from build123d import *

# Parameters (mm, degrees)
SKETCH1_W                                    = 147
SKETCH1_H                                    = 50
BOSS_EXTRUDE1_DEPTH                          = 30
FILLET1_R                                    = 10
SHELL1_T                                     = -3
CUT_EXTRUDE1_DEPTH                           = 3
CSK_FOR_M4_COUNTERSUNK_FLAT_HEAD_SCR_2_COUNT = 2
CSK_FOR_M4_COUNTERSUNK_FLAT_HEAD_SCR_2_PITCH = 32
CSK_FOR_M4_COUNTERSUNK_FLAT_HEAD_SCR_3_COUNT = 2
CSK_FOR_M4_COUNTERSUNK_FLAT_HEAD_SCR_3_PITCH = 64
CUT_EXTRUDE2_REACH                           = 32
SKETCH5_R                                    = 10


with BuildPart() as part:
    # Sketch1 → Boss-Extrude1 (new body)
    with BuildSketch(Plane(origin=(0, 0, 0), x_dir=(1, 0, 0), z_dir=(0, 1, 0))):
        Rectangle(SKETCH1_W, SKETCH1_H)
    extrude(amount=BOSS_EXTRUDE1_DEPTH)

    # Fillet1
    fillet1_edges = [part.edges().sort_by_distance(p)[0] for p in [
        (0, 0, -25),
        (0, 30, -25),
    ]]
    fillet(fillet1_edges, radius=FILLET1_R)

    # Shell1
    shell1_openings = [part.faces().sort_by_distance(p)[0] for p in [
        (0, 15, 25),
    ]]
    offset(amount=SHELL1_T, openings=shell1_openings, kind=Kind.INTERSECTION)

    # Sketch2 → Cut-Extrude1 (cut)
    with BuildSketch(Plane(origin=(0, 30, 0), x_dir=(1, 0, 0), z_dir=(0, 1, 0))):
        with BuildLine():
            Line((-70.5, -25), (-70.5, 5))
            ThreePointArc((-70.5, 5), (-67.5, 8), (-64.5, 5))
            Line((-64.5, 5), (-64.5, -25))
            Line((-64.5, -25), (-70.5, -25))
        make_face()
    cut_extrude1 = extrude(amount=-CUT_EXTRUDE1_DEPTH, mode=Mode.SUBTRACT)

    # Mirror1: Cut-Extrude1 across plane
    add(cut_extrude1.mirror(Plane(origin=(0, 0, 0), x_dir=(0, 0, 1), z_dir=(1, 0, 0))), mode=Mode.SUBTRACT)

    # Sketch3 → CSK for M4 Countersunk Flat Head Screw1 (revolve, cut)
    with BuildSketch(Plane(origin=(-32, 27, 0), x_dir=(0, 0, -1), z_dir=(1, 0, 0))):
        Polygon((0, 0), (0, 3), (2.25, 3), (2.25, 2.45), (4.7, 0), align=None)
    csk_for_m4_countersunk_flat_head_screw1 = revolve(axis=Axis((-32, 20.65, 0), (0, 1, 0)), mode=Mode.SUBTRACT)

    # CSK for M4 Countersunk Flat Head Scr 2: CSK for M4 Countersunk Flat Head Screw1 ×2
    with Locations(*[(i * CSK_FOR_M4_COUNTERSUNK_FLAT_HEAD_SCR_2_PITCH, 0, 0) for i in range(1, CSK_FOR_M4_COUNTERSUNK_FLAT_HEAD_SCR_2_COUNT)]):
        add(csk_for_m4_countersunk_flat_head_screw1, mode=Mode.SUBTRACT)

    # CSK for M4 Countersunk Flat Head Scr 3: CSK for M4 Countersunk Flat Head Screw1 ×2
    with Locations(*[(i * CSK_FOR_M4_COUNTERSUNK_FLAT_HEAD_SCR_3_PITCH, 0, 0) for i in range(1, CSK_FOR_M4_COUNTERSUNK_FLAT_HEAD_SCR_3_COUNT)]):
        add(csk_for_m4_countersunk_flat_head_screw1, mode=Mode.SUBTRACT)

    # Sketch5 → Cut-Extrude2 (cut, up to next)
    with BuildSketch(Plane.XZ, mode=Mode.PRIVATE) as cut_extrude2_sk1:
        Circle(SKETCH5_R)
    cut_extrude2_tool1 = extrude(cut_extrude2_sk1.sketch, amount=-CUT_EXTRUDE2_REACH, mode=Mode.PRIVATE) & part.part
    add(cut_extrude2_tool1.solids().sort_by_distance((0, 0, 0))[0], mode=Mode.SUBTRACT)
    # Sketch5 → Cut-Extrude2 (cut, up to next)
    with BuildSketch(Plane.XZ, mode=Mode.PRIVATE) as cut_extrude2_sk2:
        with Locations((-32, 0)):
            Circle(SKETCH5_R)
    cut_extrude2_tool2 = extrude(cut_extrude2_sk2.sketch, amount=-CUT_EXTRUDE2_REACH, mode=Mode.PRIVATE) & part.part
    add(cut_extrude2_tool2.solids().sort_by_distance((-32, 0, 0))[0], mode=Mode.SUBTRACT)
    # Sketch5 → Cut-Extrude2 (cut, up to next)
    with BuildSketch(Plane.XZ, mode=Mode.PRIVATE) as cut_extrude2_sk3:
        with Locations((32, 0)):
            Circle(SKETCH5_R)
    cut_extrude2_tool3 = extrude(cut_extrude2_sk3.sketch, amount=-CUT_EXTRUDE2_REACH, mode=Mode.PRIVATE) & part.part
    add(cut_extrude2_tool3.solids().sort_by_distance((32, 0, 0))[0], mode=Mode.SUBTRACT)


solid = part.part
Work out the finished part from the listing and answer in its coordinate system (mm). A direction names the side the tool comes from. Give positions to 0.01 mm unless a question says otherwise; leave off trailing zeros. Write each loop counter-clockwise with the first axis right and the second up, starting at its lowest first coordinate (ties: lowest second). Pieces come first, ordered by that corner, then holes.
Q1. The part is cut by section C-C on x = 67.5. Give the vertices of the cut face in (y, z), and give its area (3 significant figures).
Answer:
outline: (0, -15) arc R10 ccw to (10, -25) - (20, -25) arc R10 ccw to (30, -15) - (30, -8) - (27, -8) - (27, -15) arc R7 cw to (20, -22) - (10, -22) arc R7 cw to (3, -15) - (3, 25) - (0, 25) - close
area: 251 mm2
Q2. The part is cut by section A-A on x = 32. Give the vertices of the cut face in (y, z), and give its area (3 significant figures).
Answer:
outline: (0, -15) arc R10 ccw to (10, -25) - (20, -25) arc R10 ccw to (30, -15) - (30, -2.25) - (29.45, -2.25) - (27, -4.7) - (27, -15) arc R7 cw to (20, -22) - (10, -22) arc R7 cw to (3, -15) - (3, -10) - (0, -10) - close; (0, 10) - (3, 10) - (3, 25) - (0, 25) - close; (27, 4.7) - (29.45, 2.25) - (30, 2.25) - (30, 25) - (27, 25) - close
area: 271 mm2
Q3. The part is cut by section B-B on z = 0. State how many separate pieces and enclosed holes the cut face has, and give its area (3 significant figures).
Answer:
separate pieces: 8
enclosed holes: 0
area: 751 mm2
Q4. The part is cut by section D-D on y = 14.5. Give the vertices of the cut face in (x, z), and give its area (3 significant figures).
Answer:
outline: (-73.5, -25) - (73.5, -25) - (73.5, 25) - (70.5, 25) - (70.5, -22) - (-70.5, -22) - (-70.5, 25) - (-73.5, 25) - close
area: 723 mm2
Q5. For a pull along X with two mould halves and no side action, classify faces 5 (the face through (1.03, 26.99, -22.15)), 6 (the face through (34.13, 29.3, -1.11)), 7 (the face through (1, 24.9, -20)), 8 (the face through (73.5, 15, 0)) as released by +X, released by -X, zero draft, split by the parting line, or undercut.
Answer:
face 5: zero draft
face 6: undercut
face 7: undercut
face 8: released by +X
Q6. A tool of negligible diameter and unlimited length cuts with its end or side. For faces 1 (the face through (1, 5.1, -20)), 2 (the face through (41.54, 1.48, 3)), 3 (the face through (-67.6, 28.5, -8)), 4 (the face through (-73.5, 15, 0)), from which of +Z, -Z, +X, -X, +Y, -Y can it reach the whole face along a straight path? Write none if from no direction.
Answer:
face 1: +Z
face 2: -Y
face 3: +Z, +Y
face 4: +Z, -Z, -X, +Y, -Y
Q7. Given pin 1 (2 mm diameter, centred on x = -25, y = 24.5, fed in from +Z); pin 2 (6 mm diameter, centred on x = 32, z = 0, fed in from -Y); pin 3 (8 mm diameter, centred on x = 22, y = 17, fed in from +Z), each flat-ended and moving along its own axis, determine where each tip first touches the part or whether it passes through.
Answer:
pin 1: stops at z = -19.33
pin 2: stops at y = 28.7
pin 3: stops at z = -21.93
Q8. Straight lines are drawn through the part: L1, parallel to X at y = 29.9, z = 0; L2, parallel to Y at x = 27.5, z = 18; L3, parallel to X at y = 4.75, z = -8.5. For each, find the intervals that lie inside material, in ascending order.
Answer:
L1: x = -73.5 to -70.5, -64.5 to -34.25, -29.75 to -2.25, 2.25 to 29.75, 34.25 to 64.5, 70.5 to 73.5
L2: y = 0 to 3, 27 to 30
L3: x = -73.5 to -70.5, 70.5 to 73.5
